from build123d import *

# Parameters (mm, degrees)
SKETCH1_R             = 18
BOSS_EXTRUDE1_DEPTH   = 2
SKETCH2_R             = 1.6
CUT_EXTRUDE1_DEPTH    = 2
F_2_0MM_DOWEL_HOLE1_D = 2
SKETCH5_R             = 1.6
CUT_EXTRUDE4_DEPTH    = 44.603325561
FILLET1_R             = 4


with BuildPart() as part:
    # Sketch1 → Boss-Extrude1 (new body)
    with BuildSketch(Plane.XY):
        with BuildLine():
            Line((-32.5, 20.5), (-20.512191497, 20.5))
            ThreePointArc((-20.512191497, 20.5), (0, 29), (20.512191497, 20.5))
            Line((20.512191497, 20.5), (32.5, 20.5))
            Line((32.5, 20.5), (32.5, -20.5))
            Line((32.5, -20.5), (20.512191497, -20.5))
            ThreePointArc((20.512191497, -20.5), (0, -29), (-20.512191497, -20.5))
            Line((-20.512191497, -20.5), (-32.5, -20.5))
            Line((-32.5, -20.5), (-32.5, 20.5))
        make_face()
        Circle(SKETCH1_R, mode=Mode.SUBTRACT)
    extrude(amount=BOSS_EXTRUDE1_DEPTH)

    # Sketch2 → Cut-Extrude1 (cut)
    with BuildSketch(Plane.XY.offset(2)):
        with Locations((-29, 14)):
            Circle(SKETCH2_R)
        with Locations((-29, -18)):
            Circle(SKETCH2_R)
        with Locations((29, -18)):
            Circle(SKETCH2_R)
        with Locations((29, 14)):
            Circle(SKETCH2_R)
    extrude(amount=-CUT_EXTRUDE1_DEPTH, mode=Mode.SUBTRACT)

    # Ø2.0mm Dowel Hole1 (through all)
    with Locations(Plane(origin=(-19, 19, 2), x_dir=(1, 0, 0), z_dir=(0, 0, 1))):
        with Locations((0, 0), (2, -2), (36, -2), (38, 0), (36, -36), (38, -38), (0, -38), (2, -36)):
            Hole(F_2_0MM_DOWEL_HOLE1_D / 2)

    # Sketch5 → Cut-Extrude4 (cut, through all)
    with BuildSketch(Plane.XY):
        with Locations((0, 25)):
            Circle(SKETCH5_R)
        with Locations((-25, 0)):
            Circle(SKETCH5_R)
        with Locations((25, 0)):
            Circle(SKETCH5_R)
        with Locations((0, -25)):
            Circle(SKETCH5_R)
    extrude(amount=CUT_EXTRUDE4_DEPTH, mode=Mode.SUBTRACT)

    # Fillet1
    fillet1_edges = [part.edges().sort_by_distance(p)[0] for p in [
        (-32.5, -20.5, 1),
        (-32.5, 20.5, 1),
        (32.5, 20.5, 1),
        (32.5, -20.5, 1),
    ]]
    fillet(fillet1_edges, radius=FILLET1_R)


solid = part.part
Source: CAD feature listing. Evaluate the final solid. Frame: model axes, mm. A direction names the side the tool comes from. Round coordinates to 2 decimals unless told otherwise and drop trailing zeros. Loops run counter-clockwise (first coordinate to the right, second up) from the corner with the lowest first, then second, coordinate; pieces in that order, holes last. Notation, with made-up numbers: M 80,14 L 99,14 A37 ccw 99,52 Z; hole C 2.25,39.5 d2. An arc over 180 degrees is marked long. Return JSON: item names as keys, results as strings. Group by question number.
1. Pin query (flat end, axial travel): pin 1 (2.5 mm diameter, centred on x = 25, y = 0, fed in from -Z). Return the tip coordinate at first contact, or that it passes through.
2. Reachability of faces 1 (the face through (-25, 20.5, 1)), 2 (the face through (17, 16, 1)) from +Z, -Z, +X, -X, +Y, -Y: full face, straight path, thin tool, end or side. Return the list, or none.
3. Section query C-C on x = -19. Output: boundary loops of the cut face in (y, z), and give its area (3 significant figures).
4. Section query B-B on y = 0. Output: boundary loops of the cut face in (x, z).
5. Section query D-D on y = -14. Output: boundary loops of the cut face in (x, z).
6. Mould query, pull axis Y, two halves, no side actions, for faces 3 (the face through (0, 29, 1)), 4 (the face through (-29.208, -16.414, 1.014)), 5 (the face through (-24, -20.5, 1)). Classes: released by +Y, released by -Y, zero draft, split by the parting line, or undercut.
7. Section query A-A on z = 1.45. State how many separate pieces and enclosed holes the cut face has, and give its area (3 significant figures).
8. Material intervals for line 1 along Y through (x, z) = (-19, 1.2); line 2 along Y through (x, z) = (-25, 1.4); line 3 along Y through (x, z) = (21.5, 1.25), sorted ascending. Write a range as from..to.
Checks:
{
 "1": {"pin 1": "passes through"},
 "2": {"face 1": "+Z, -Z, -X, +Y", "face 2": "+Z, -Z"},
 "3": {"outline": "M -21.91,0 L -20,0 L -20,2 L -21.91,2 Z; M -18,0 L 18,0 L 18,2 L -18,2 Z; M 20,0 L 21.91,0 L 21.91,2 L 20,2 Z", "area": "79.6 mm²"},
 "4": {"outline": "M -32.5,0 L -26.6,0 L -26.6,2 L -32.5,2 Z; M -23.4,0 L -18,0 L -18,2 L -23.4,2 Z; M 18,0 L 23.4,0 L 23.4,2 L 18,2 Z; M 26.6,0 L 32.5,0 L 32.5,2 L 26.6,2 Z"},
 "5": {"outline": "M -32.5,0 L -11.31,0 L -11.31,2 L -32.5,2 Z; M 11.31,0 L 32.5,0 L 32.5,2 L 11.31,2 Z"},
 "6": {"face 3": "released by +Y", "face 4": "undercut", "face 5": "released by -Y"},
 "7": {"separate pieces": "1", "enclosed holes": "17", "area": "2,020 mm²"},
 "8": {"line 1": "y = -21.91..-20, -18..18, 20..21.91", "line 2": "y = -20.5..-1.6, 1.6..20.5", "line 3": "y = -20.5..20.5"}
}
